Here's how the part is built. I have some questions about the finished solid (model axes, mm). Face numbers are marked on the shaded views. A direction names the side the tool comes from. Coordinates: 2 decimals unless noted, no trailing zeros. Loops run counter-clockwise (first coordinate to the right, second up) from the corner with the lowest first, then second, coordinate; pieces in that order, holes last.
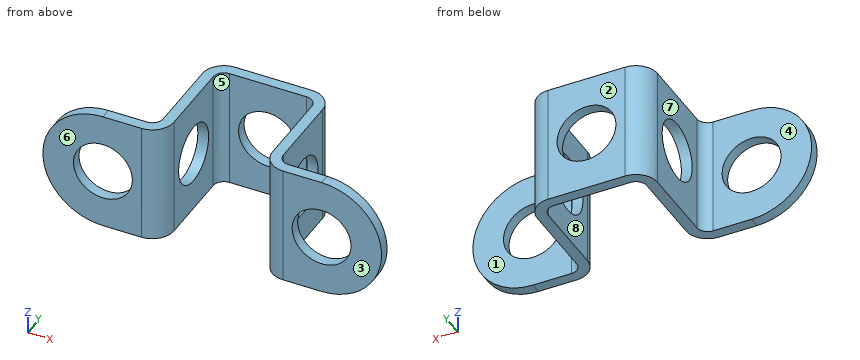
from build123d import *

# Parameters (mm, degrees)
SKETCH1_W                      = 10
SKETCH1_H                      = 10
SKETCH1_R                      = 2.45
BASE_FLANGE1_DEPTH             = 0.9
EDGE_FLANGE1_STRIP_W           = 5.4
EDGE_FLANGE1_STRIP_H           = 0.9
EDGE_FLANGE1_STRIP_CUT_DEPTH   = 10
EDGE_FLANGE1_STRIP_2_W         = 5.4
EDGE_FLANGE1_STRIP_2_H         = 0.9
EDGE_FLANGE1_STRIP_CUT_2_DEPTH = 10
EDGE_FLANGE1_DEPTH             = 10
EDGE_FLANGE1_BEND_DEPTH        = 10
EDGE_FLANGE2_STRIP_W           = 5.4
EDGE_FLANGE2_STRIP_H           = 0.9
EDGE_FLANGE2_STRIP_CUT_DEPTH   = 10
EDGE_FLANGE2_STRIP_2_W         = 5.4
EDGE_FLANGE2_STRIP_2_H         = 0.9
EDGE_FLANGE2_STRIP_CUT_2_DEPTH = 10
EDGE_FLANGE2_DEPTH             = 10
EDGE_FLANGE2_BEND_DEPTH        = 10
HOLE1_OUTLINE_R                = 2.45
HOLE1_DEPTH                    = 10
SKETCH21_R                     = 2.45
CUT_EXTRUDE1_DEPTH             = 10


# Read off the part's stored shape, not the designer's step: Hole1
# Sheet-metal steps are written as plain solids
with BuildPart() as part:
    # Sketch1 → Base-Flange1 (new body)
    with BuildSketch(Plane(origin=(0, 0, 0), x_dir=(1, 0, 0), z_dir=(0, 1, 0))):
        with Locations((5, 5)):
            Rectangle(SKETCH1_W, SKETCH1_H)
        with Locations(Location((5, 5, 0), (0, 0, 270))):
            Circle(SKETCH1_R, mode=Mode.SUBTRACT)
    extrude(amount=-BASE_FLANGE1_DEPTH)

    # Edge-Flange1 strip (across the edge) → Edge-Flange1 strip cut (cut)
    with BuildSketch(Plane(origin=(10, -0.9, -10), x_dir=(-1, 0, 0), z_dir=(0, 0, 1))):
        with Locations((-0.9, -0.45)):
            Rectangle(EDGE_FLANGE1_STRIP_W, EDGE_FLANGE1_STRIP_H)
    extrude(amount=EDGE_FLANGE1_STRIP_CUT_DEPTH, mode=Mode.SUBTRACT)

    # Edge-Flange1 strip 2 (across the edge) → Edge-Flange1 strip cut 2 (cut)
    with BuildSketch(Plane(origin=(0, -0.9, 0), x_dir=(1, 0, 0), z_dir=(0, 0, -1))):
        with Locations((-0.9, -0.45)):
            Rectangle(EDGE_FLANGE1_STRIP_2_W, EDGE_FLANGE1_STRIP_2_H)
    extrude(amount=EDGE_FLANGE1_STRIP_CUT_2_DEPTH, mode=Mode.SUBTRACT)

    # Edge-Flange1 section (across the edge) → Edge-Flange1 (add)
    with BuildSketch(Plane(origin=(10, -0.9, -10), x_dir=(-1, 0, 0), z_dir=(0, 0, 1))):
        with BuildLine():
            Line((0, 0.9), (0, 9.1))
            Line((0, 9.1), (0.9, 9.1))
            Line((0.9, 9.1), (0.9, 0.9))
            ThreePointArc((0.9, 0.9), (1.163603897, 0.263603897), (1.8, 0))
            Line((1.8, 0), (1.8, -0.9))
            ThreePointArc((1.8, -0.9), (0.527207794, -0.372792206), (0, 0.9))
        make_face()
    extrude(amount=EDGE_FLANGE1_DEPTH)

    # Edge-Flange1 section 2 (across the edge) → Edge-Flange1 bend (add)
    with BuildSketch(Plane(origin=(0, -0.9, 0), x_dir=(1, 0, 0), z_dir=(0, 0, -1))):
        with BuildLine():
            Line((0, 0.9), (0, 9.1))
            Line((0, 9.1), (0.9, 9.1))
            Line((0.9, 9.1), (0.9, 0.9))
            ThreePointArc((0.9, 0.9), (1.163603897, 0.263603897), (1.8, 0))
            Line((1.8, 0), (1.8, -0.9))
            ThreePointArc((1.8, -0.9), (0.527207794, -0.372792206), (0, 0.9))
        make_face()
    extrude(amount=EDGE_FLANGE1_BEND_DEPTH)

    # Edge-Flange2 strip (across the edge) → Edge-Flange2 strip cut (cut)
    with BuildSketch(Plane(origin=(10, -10, 0), x_dir=(0, 1, 0), z_dir=(0, 0, -1))):
        with Locations((-0.9, -0.45)):
            Rectangle(EDGE_FLANGE2_STRIP_W, EDGE_FLANGE2_STRIP_H)
    extrude(amount=EDGE_FLANGE2_STRIP_CUT_DEPTH, mode=Mode.SUBTRACT)

    # Edge-Flange2 strip 2 (across the edge) → Edge-Flange2 strip cut 2 (cut)
    with BuildSketch(Plane(origin=(0, -10, -10), x_dir=(0, 1, 0), z_dir=(0, 0, 1))):
        with Locations((-0.9, -0.45)):
            Rectangle(EDGE_FLANGE2_STRIP_2_W, EDGE_FLANGE2_STRIP_2_H)
    extrude(amount=EDGE_FLANGE2_STRIP_CUT_2_DEPTH, mode=Mode.SUBTRACT)

    # Edge-Flange2 section (across the edge) → Edge-Flange2 (add)
    with BuildSketch(Plane(origin=(10, -10, 0), x_dir=(0, 1, 0), z_dir=(0, 0, -1))):
        with BuildLine():
            Line((0, 0.9), (0, 9.1))
            Line((0, 9.1), (0.9, 9.1))
            Line((0.9, 9.1), (0.9, 0.9))
            ThreePointArc((0.9, 0.9), (1.163603897, 0.263603897), (1.8, 0))
            Line((1.8, 0), (1.8, -0.9))
            ThreePointArc((1.8, -0.9), (0.527207794, -0.372792206), (0, 0.9))
        make_face()
    extrude(amount=EDGE_FLANGE2_DEPTH)

    # Edge-Flange2 section 2 (across the edge) → Edge-Flange2 bend (add)
    with BuildSketch(Plane(origin=(0, -10, -10), x_dir=(0, 1, 0), z_dir=(0, 0, 1))):
        with BuildLine():
            Line((0, 0.9), (0, 9.1))
            Line((0, 9.1), (0.9, 9.1))
            Line((0.9, 9.1), (0.9, 0.9))
            ThreePointArc((0.9, 0.9), (1.163603897, 0.263603897), (1.8, 0))
            Line((1.8, 0), (1.8, -0.9))
            ThreePointArc((1.8, -0.9), (0.527207794, -0.372792206), (0, 0.9))
        make_face()
    extrude(amount=EDGE_FLANGE2_BEND_DEPTH)

    # Hole1 outline → Hole1 (cut)
    with BuildSketch(Plane.YZ):
        with Locations((-5, -5)):
            Circle(HOLE1_OUTLINE_R)
    extrude(amount=HOLE1_DEPTH, mode=Mode.SUBTRACT)

    # Sketch21 → Cut-Extrude1 (cut)
    with BuildSketch(Plane(origin=(0, -9.1, 0), x_dir=(1, 0, 0), z_dir=(0, 1, 0))):
        with Locations(Location((14.1, 5, 0), (0, 0, 270))):
            Circle(SKETCH21_R)
        with Locations(Location((-4.1, 5, 0), (0, 0, 90))):
            Circle(SKETCH21_R)
        with BuildLine():
            Line((-4.1, 10), (-4.552354971, 12.340568082))
            Line((-4.552354971, 12.340568082), (-11.187715638, 12.084129022))
            Line((-11.187715638, 12.084129022), (-11.412099815, 3.1728717))
            Line((-11.412099815, 3.1728717), (-10.931276579, -1.41097649))
            Line((-10.931276579, -1.41097649), (-3.526598732, -3.206049908))
            Line((-3.526598732, -3.206049908), (-4.1, 0))
            ThreePointArc((-4.1, 0), (-9.1, 5), (-4.1, 10))
        make_face()
        with BuildLine():
            Line((14.1, 10), (20.065794752, 12.917555966))
            Line((20.065794752, 12.917555966), (23.30333788, -2.532897376))
            Line((23.30333788, -2.532897376), (14.680574501, -2.532897376))
            Line((14.680574501, -2.532897376), (14.1, 0))
            ThreePointArc((14.1, 0), (19.1, 5), (14.1, 10))
        make_face()
    extrude(amount=-CUT_EXTRUDE1_DEPTH, mode=Mode.SUBTRACT)


solid = part.part
Q1. Please list where these lines run through material, in increasing order: probe 1 along X at (y, z) = (-3.25, -3); probe 2 along Z at (x, y) = (0.3, -5); probe 3 along Y at (x, z) = (15.75, -0.75).
Q2. We'd pull the mould along X, two halves only. Please class the marked faces 6, 7 and 8: pulls with the +X half, pulls with the -X half, needs draft (parallel to the pull), parting line crosses it, or undercut.
Q3. Will these pins go through, and if not, where does the flat tip stop? P1, Ø4, axis at x = 2, z = -8.5, coming from the -Y side; P2, Ø1.9, axis at y = -5.5, z = -3.5, coming from the +X side; P3, Ø4, axis at x = -5.5, z = -3.5, coming from the +Y side.
Q4. Suppose I cut it at B-B on x = 5. Write out the boundary of the cut face in (y, z).
Q5. Suppose I cut it at D-D on z = -2. Write out the boundary of the cut face in (x, y).
Q6. Suppose I cut it at C-C on y = -7.75. Write out the boundary of the cut face in (x, z).
Q7. For the marked faces 1, 2, 3, 4 and 5, which set-ups out of +Z, -Z, +X, -X, +Y, -Y let a thin tool reach every point of the face, with its end or its side?
Q8. Suppose I cut it at A-A on y = -5. Write out the boundary of the cut face in (x, z).
Check values:
1. probe 1: x = 0 to 0.9, 9.1 to 10
1. probe 2: z = -10 to -7.45, -2.55 to 0
1. probe 3: y = -10 to -9.1
2. face 6: needs draft
2. face 7: pulls with the -X half
2. face 8: undercut
3. P1: stops at y = -9.76
3. P2: stops at x = 10
3. P3: stops at y = -9.1
4. outline: (-0.9, -10) - (0, -10) - (0, -7.45) - (-0.9, -7.45) - close; (-0.9, -2.55) - (0, -2.55) - (0, 0) - (-0.9, 0) - close
5. outline: (-8.1, -10) - (-0.9, -10) arc R1.8 ccw to (0.9, -8.2) - (0.9, -1.8) arc R0.9 cw to (1.8, -0.9) - (8.2, -0.9) arc R0.9 cw to (9.1, -1.8) - (9.1, -8.2) arc R1.8 ccw to (10.9, -10) - (18.1, -10) - (18.1, -9.1) - (10.9, -9.1) arc R0.9 cw to (10, -8.2) - (10, -1.8) arc R1.8 ccw to (8.2, 0) - (1.8, 0) arc R1.8 ccw to (0, -1.8) - (0, -8.2) arc R0.9 cw to (-0.9, -9.1) - (-8.1, -9.1) - close
6. outline: (0, -10) - (0.9, -10) - (0.9, 0) - (0, 0) - close; (9.1, -10) - (10, -10) - (10, 0) - (9.1, 0) - close
7. face 1: +Z, -Z, +X, +Y
7. face 2: +Z, -Z, +X, -X, +Y
7. face 3: +Z, -Z, +X, -X, -Y
7. face 4: +Z, -Z, -X, +Y
7. face 5: +Z, -Z, -Y
8. outline: (0, -10) - (0.9, -10) - (0.9, -7.45) - (0, -7.45) - close; (0, -2.55) - (0.9, -2.55) - (0.9, 0) - (0, 0) - close; (9.1, -10) - (10, -10) - (10, -7.45) - (9.1, -7.45) - close; (9.1, -2.55) - (10, -2.55) - (10, 0) - (9.1, 0) - close
